Geometry: see drawing. Coordinates: mm, zero at the bounding-box minimum. A direction names the side the tool comes from. Give positions to 0.01 mm unless a question says otherwise; leave off trailing zeros. Loops run counter-clockwise (first coordinate to the right, second up) from the corner with the lowest first, then second, coordinate; pieces in that order, holes last. Notation, with made-up numbers: M 70,34 L 89,34 A27 ccw 89,54 Z; hole C 3.25,53 d3. An arc over 180 degrees is marked long. Put each result on its own line as item: value.
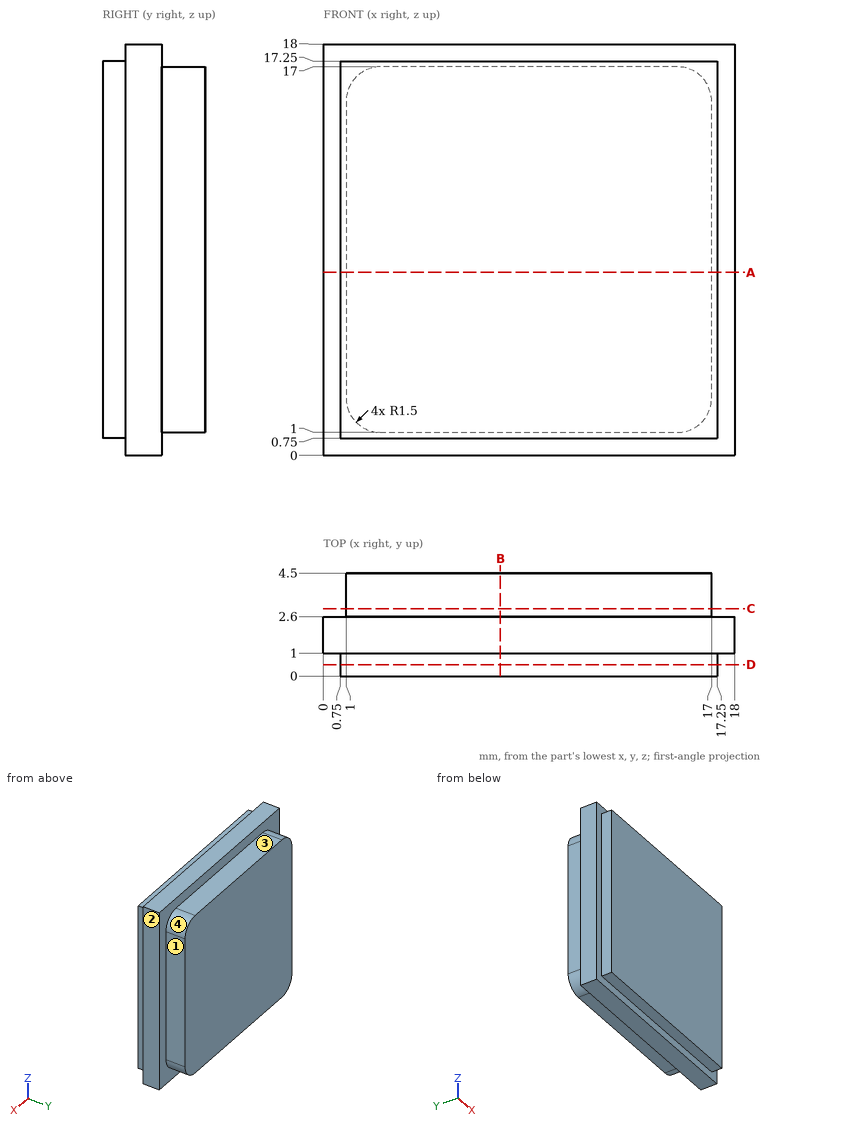
Item 1: Pin query (flat end, axial travel): pin 1 Ø0.6 at (x, y) = (6.5, 3.5) entering from -Z; pin 2 Ø0.6 at (y, z) = (3.5, 11) entering from +X; pin 3 Ø0.5 at (x, y) = (6.5, 0.5) entering from -Z. Return the tip coordinate at first contact, or that it passes through.
Output values:
pin 1: z = 1
pin 2: x = 17
pin 3: z = 0.75
Item 2: Section A-A on z = 8. Output: boundary loops of the cut face in (x, y), then the cut area to 3 significant figures.
Output values:
outline: M 0,1 L 0.75,1 L 0.75,0 L 17.25,0 L 17.25,1 L 18,1 L 18,2.6 L 17,2.6 L 17,4.5 L 1,4.5 L 1,2.6 L 0,2.6 Z
area: 75.7 mm²
Item 3: Section D-D on y = 0.5. Output: boundary loops of the cut face in (x, z).
Output values:
outline: M 0.75,0.75 L 17.25,0.75 L 17.25,17.25 L 0.75,17.25 Z
Item 4: Line query: probe 1 along Z at (x, y) = (5.75, 3.9); probe 2 along X at (y, z) = (0.95, 14.75). Output: solid intervals per line, ascending. Write a range as [from, to].
Output values:
probe 1: [1, 17]
probe 2: [0.75, 17.25]
Item 5: Section B-B on x = 7.75. Output: boundary loops of the cut face in (y, z).
Output values:
outline: M 0,0.75 L 1,0.75 L 1,0 L 2.6,0 L 2.6,1 L 4.5,1 L 4.5,17 L 2.6,17 L 2.6,18 L 1,18 L 1,17.25 L 0,17.25 Z
Item 6: Section C-C on y = 2.95. Output: boundary loops of the cut face in (x, z).
Output values:
outline: M 1,2.5 A1.5 ccw 2.5,1 L 15.5,1 A1.5 ccw 17,2.5 L 17,15.5 A1.5 ccw 15.5,17 L 2.5,17 A1.5 ccw 1,15.5 Z
Item 7: Set-up query: the marked faces 1, 2, 3 and 4. Return all of +Z, -Z, +X, -X, +Y, -Y with unobstructed straight access to the full face (end or side cutting, diameter ignored); none if empty.
Output values:
face 1: +Z, -Z, +X, +Y
face 2: +Z, -Z, +X, +Y, -Y
face 3: +Z, +X, -X, +Y
face 4: +Z, +X, +Y
